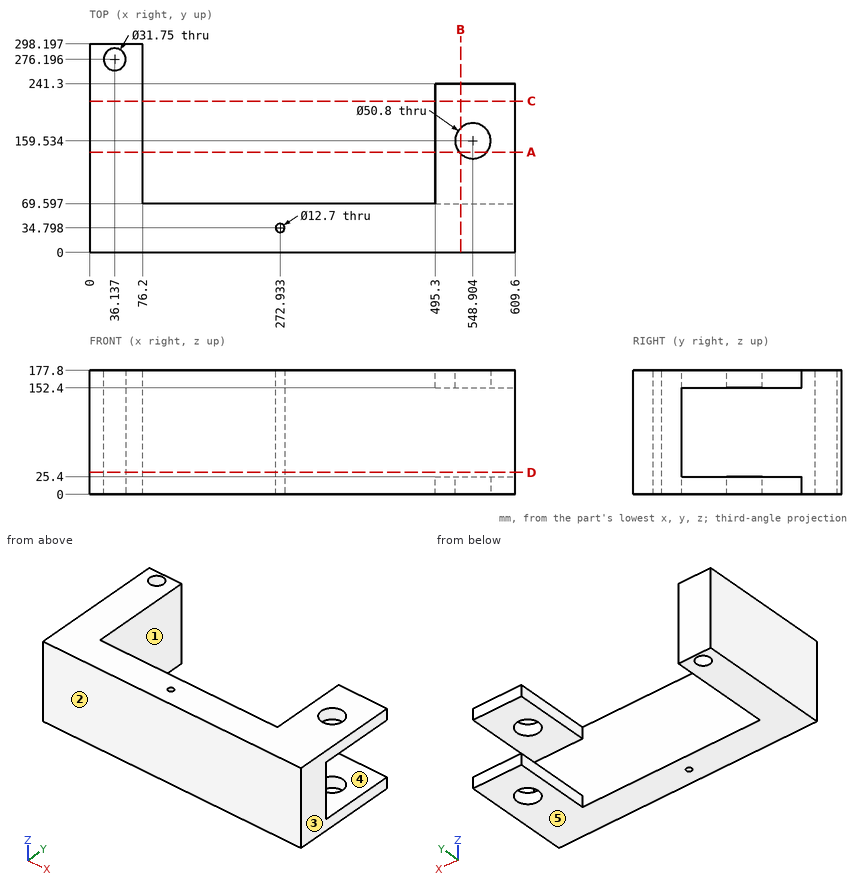
Geometry check sheet. Reference: drawing and pictorial views, mm from the part's lowest x, y, z. A direction names the side the tool comes from. Round coordinates to 2 decimals unless told otherwise and drop trailing zeros. Order: outer loops, then holes, each group sorted by start corner. A loop starts at its lowest first (then second) coordinate and runs counter-clockwise, first axis right, second up. Notation, with made-up numbers: (-32, -19) - (7, -19) arc R14 cw to (7, -12) - close; hole circle Ø11 at (-30, 14.5). An arc over 180 degrees is marked (long way). Use a Markdown table: item, result. Add a question column.
1) Section check B-B (x = 531.5). Record the cut outline in (y, z) (1 decimal), then the cut area to 3 significant figures.
2) Thickness scan on line 1 along X through (y, z) = (75, 90.5); line 2 along X through (y, z) = (234, 20.5); line 3 along Y through (x, z) = (116.5, 10.5). Record the ranges inside material, lowest first.
3) Section check A-A (y = 143.5). Record the cut outline in (x, z) (1 decimal), then the cut area to 3 significant figures.
4) Gauge pin test, flat ends, axial feed: P1, Ø3, axis at y = 220, z = 137.5, coming from the +X side; P2, Ø20.5, axis at x = 544.5, z = 164.5, coming from the +Y side; P3, Ø12, axis at x = 472.5, z = 137, coming from the +Y side. Record the tip position at first contact, or that the pin passes through.
5) Section check D-D (z = 31.5). Count the separate pieces of the cut face and the enclosed holes in it, then the cut area to 3 significant figures.
6) Set-up check for the marked faces 4 and 5: record each of +Z, -Z, +X, -X, +Y, -Y from which the full face is reachable in a straight line by a thin tool's end or side.
7) Section check C-C (y = 216.5). Record the cut outline in (x, z).
8) Mould release check, pull along X, two halves, no side actions. Record for the marked faces 1, 2 and 3: released by +X, released by -X, zero draft, split by the parting line, or undercut.
Established:
| question | item | result |
|---|---|---|
| 1 | outline | (0, 0) - (141, 0) - (141, 25.4) - (69.6, 25.4) - (69.6, 152.4) - (141, 152.4) - (141, 177.8) - (0, 177.8) - close; (178, 0) - (241.3, 0) - (241.3, 25.4) - (178, 25.4) - close; (178, 152.4) - (241.3, 152.4) - (241.3, 177.8) - (178, 177.8) - close |
| 1 | area | 19,200 mm2 |
| 2 | line 1 | 0 to 76.2 |
| 2 | line 2 | 0 to 76.2, 495.3 to 609.6 |
| 2 | line 3 | 0 to 69.6 |
| 3 | outline | (0, 0) - (76.2, 0) - (76.2, 177.8) - (0, 177.8) - close; (495.3, 0) - (529.2, 0) - (529.2, 25.4) - (495.3, 25.4) - close; (495.3, 152.4) - (529.2, 152.4) - (529.2, 177.8) - (495.3, 177.8) - close; (568.6, 0) - (609.6, 0) - (609.6, 25.4) - (568.6, 25.4) - close; (568.6, 152.4) - (609.6, 152.4) - (609.6, 177.8) - (568.6, 177.8) - close |
| 3 | area | 17,400 mm2 |
| 4 | P1 | x = 76.2 |
| 4 | P2 | y = 241.3 |
| 4 | P3 | y = 69.6 |
| 5 | separate pieces | 1 |
| 5 | enclosed holes | 2 |
| 5 | area | 58,900 mm2 |
| 6 | face 4 | +X, +Y |
| 6 | face 5 | -Z, +X, -X, +Y, -Y |
| 7 | outline | (0, 0) - (76.2, 0) - (76.2, 177.8) - (0, 177.8) - close; (495.3, 0) - (609.6, 0) - (609.6, 25.4) - (495.3, 25.4) - close; (495.3, 152.4) - (609.6, 152.4) - (609.6, 177.8) - (495.3, 177.8) - close |
| 8 | face 1 | undercut |
| 8 | face 2 | zero draft |
| 8 | face 3 | released by +X |
